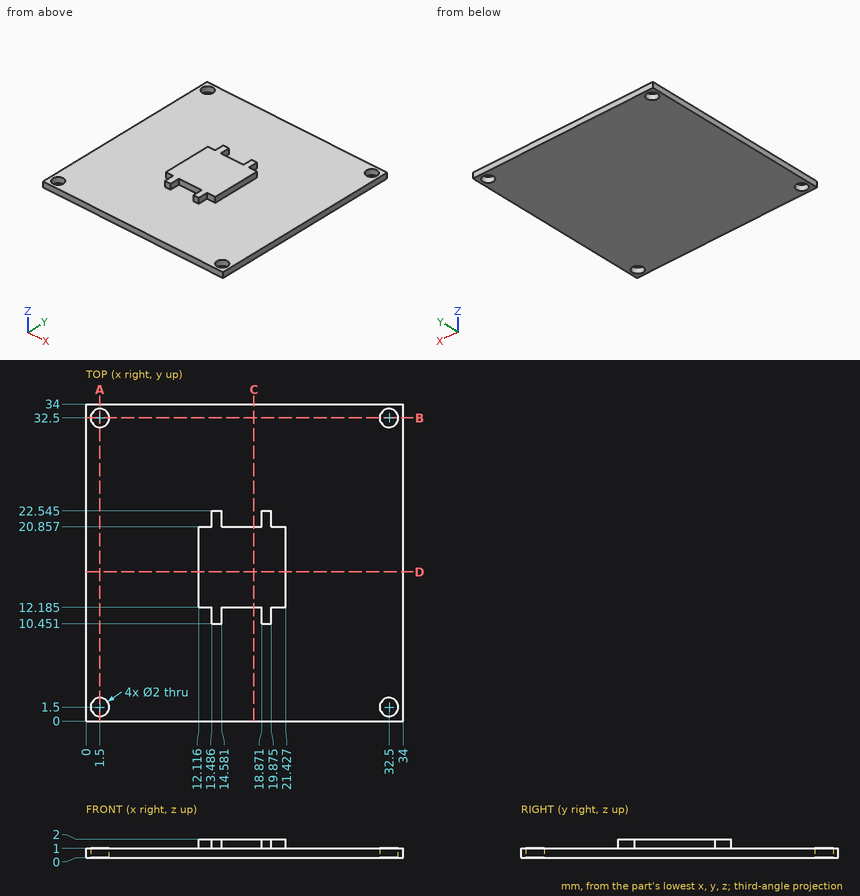
Here's the drawing with two shaded views (mm, measured from the low corner). I have some questions. Coordinates: 2 decimals unless noted, no trailing zeros. Order: outer loops, then holes, each group sorted by start corner. A loop starts at its lowest first (then second) coordinate and runs counter-clockwise, first axis right, second up. Notation, with made-up numbers: (44, 43.25) -> (58, 43.25) arc R24 cw to (58, 79.25) -> close; hole circle Ø4 at (-34, 54.5). An arc over 180 degrees is marked (long way). Write each question's results on one line, items separated by ' | '.
Item 1: I want a section at A-A, the plane x = 1.5. Write out the boundary of the cut face in (y, z).
Results are:
outline: (0, 0) -> (0.5, 0) -> (0.5, 1) -> (0, 1) -> close; (2.5, 0) -> (31.5, 0) -> (31.5, 1) -> (2.5, 1) -> close; (33.5, 0) -> (34, 0) -> (34, 1) -> (33.5, 1) -> close
Item 2: I want a section at D-D, the plane y = 16. Write out the boundary of the cut face in (x, z).
Results are:
outline: (0, 0) -> (34, 0) -> (34, 1) -> (21.43, 1) -> (21.43, 2) -> (12.12, 2) -> (12.12, 1) -> (0, 1) -> close
Item 3: I want a section at C-C, the plane x = 18. Write out the boundary of the cut face in (y, z) (1 decimal).
Results are:
outline: (0, 0) -> (34, 0) -> (34, 1) -> (20.9, 1) -> (20.9, 2) -> (12.2, 2) -> (12.2, 1) -> (0, 1) -> close
Item 4: I'm going to push flat-ended pins straight in: pin 1 Ø5 at (x, y) = (21.5, 7) entering from -Z; pin 2 Ø0.8 at (y, z) = (12, 1.5) entering from -X; pin 3 Ø0.5 at (y, z) = (21.5, 1.5) entering from +X (1 decimal); pin 4 Ø0.5 at (x, z) = (20.5, 1.5) entering from +Y. Where does each tip first touch, or does it pass through?
Results are:
pin 1: z = 0 | pin 2: x = 12.12 | pin 3: x = 19.9 | pin 4: y = 20.86
Item 5: If I drill on line 1 along Y through (x, z) = (1.5, 0.3); line 2 along Y through (x, z) = (32, 0.5) (1 decimal); line 3 along Z through (x, y) = (8, 26.5), over which ranges is the centre line in solid material (lowest first)?
Results are:
line 1: 0 to 0.5, 2.5 to 31.5, 33.5 to 34 | line 2: 0 to 0.6, 2.4 to 31.6, 33.4 to 34 | line 3: 0 to 1
